Autodesk Inventor part; units mm, degrees
ref_plane "YZ Plane" through (0, 0, 0) normal (1, 0, 0) x (0, 1, 0)
ref_plane "XZ Plane" through (0, 0, 0) normal (0, 1, 0) x (-1, 0, 0)
ref_plane "XY Plane" through (0, 0, 0) normal (0, 0, 1) x (1, 0, 0)
sketch "Sketch1" plane through (0, 0, 0) normal (0, 0, 1) x (1, 0, 0)
  line L0 (-300, -400) -> (300, -400)
  line L1 (300, -400) -> (300, 400)
  line L2 (300, 400) -> (-300, 400)
  line L3 (-300, 400) -> (-300, -400)
  line L4 (-300, -400) -> (300, 400) construction
  line L5 (300, -400) -> (-300, 400) construction
  line L6 (-80, 360) -> (80, 360)
  line L7 (80, 360) -> (80, 400)
  line L8 (80, 400) -> (-80, 400)
  line L9 (-80, 400) -> (-80, 360)
  line L10 (-80, 360) -> (80, 400) construction
  line L11 (80, 360) -> (-80, 400) construction
  line L12 (-300, 280) -> (-260, 280)
  line L13 (-260, 280) -> (-180, 360)
  line L14 (-180, 360) -> (-180, 400)
  line L15 (180, 400) -> (180, 360)
  line L16 (180, 360) -> (260, 280)
  line L17 (260, 280) -> (300, 280)
  line L18 (-300, -275) -> (-260, -275)
  line L19 (-260, -275) -> (-260, -400)
  line L20 (300, -280) -> (260, -280)
  line L21 (260, -280) -> (260, -400)
  line L22 (0, 0) -> (0, 380) construction
  line L23 (-1, 360) -> (1, 360)
  line L24 (1, 360) -> (1, -400)
  line L25 (1, -400) -> (-1, -400)
  line L26 (-1, -400) -> (-1, 360)
  line L27 (-179, 400) -> (-179, 359.5858)
  line L28 (-179, 359.5858) -> (-259.5858, 279)
  line L29 (-259.5858, 279) -> (-300, 279)
  line L30 (-81, 359) -> (81, 359)
  line L31 (81, 359) -> (81, 401)
  line L32 (81, 401) -> (-81, 401)
  line L33 (-81, 401) -> (-81, 359)
  line L34 (-299, 399) -> (299, 399)
  line L35 (299, 399) -> (299, -399)
  line L36 (299, -399) -> (-299, -399)
  line L37 (-299, -399) -> (-299, 399)
  line L38 (-300, -274) -> (-259, -274)
  line L39 (-259, -274) -> (-259, -400)
  line L40 (259, -400) -> (259, -279)
  line L41 (259, -279) -> (300, -279)
  line L42 (300, 279) -> (259.5858, 279)
  line L43 (259.5858, 279) -> (179, 359.5858)
  line L44 (179, 359.5858) -> (179, 400)
  line L45 (-40, 360) -> (40, 360)
  line L46 (40, 360) -> (40, 280)
  line L47 (40, 280) -> (-40, 280)
  line L48 (-40, 280) -> (-40, 360)
  line L49 (-41, 361) -> (41, 361)
  line L50 (41, 361) -> (41, 279)
  line L51 (41, 279) -> (-41, 279)
  line L52 (-41, 279) -> (-41, 361)
  point P0 (-299, 279)
  point P1 (-299, -274)
  point P2 (-259, -399)
  point P3 (-1, -399)
  point P4 (-1, 359)
  point P5 (-81, 399)
  point P6 (-179, 399)
  point P7 (-1, 279)
  point P8 (-41, 359)
  dimension "d0" = 600
  dimension "d1" = 800
  dimension "d2" = 160
  dimension "d3" = 40
  dimension "d4" = 40
  dimension "d5" = 40
  dimension "d6" = 40
  dimension "d7" = 40
  dimension "d8" = 40
  dimension "d9" = 40
  dimension "d10" = 120
  dimension "d11" = 120
  dimension "d12" = 120
  dimension "d13" = 120
  dimension "d14" = 125
  dimension "d15" = 120
  dimension "d16" = 2
  dimension "d17" = 1
  dimension "d18" = 1
  dimension "d19" = 1
  dimension "d20" = 1
  dimension "d21" = 1
  dimension "d22" = 1
  dimension "d25" = 80
  dimension "d26" = 80
  dimension "d27" = 1
extrude "Extrusion1" add sketch "Sketch1" along normal blind 4 contours L39 L38 L37 L29 L28 L27 L34 L33 L30 L52 L51 L26 L36
fillet "Fillet1" radius 4 13 edges at (-179, 399, 2) (-179, 359.5858, 2) (-259.5858, 279, 2) (-299, 279, 2) (-81, 399, 2) (-81, 359, 2) (-41, 359, 2) (-41, 279, 2) (-1, 279, 2) (-1, -399, 2) (-259, -399, 2) (-259, -274, 2) (-299, -274, 2)
sketch "Sketch2" plane through (0, 0, 4) normal (0, 0, 1) x (1, 0, 0)
  arc A0 (-299, -270) -> (-295, -274) centre (-295, -270) ccw
  line L0 (-295, -274) -> (-263, -274)
  arc A1 (-259, -278) -> (-263, -274) centre (-263, -278) ccw
  line L1 (-259, -278) -> (-259, -395)
  arc A2 (-259, -395) -> (-255, -399) centre (-255, -395) ccw
  line L2 (-255, -399) -> (-5, -399)
  arc A3 (-5, -399) -> (-1, -395) centre (-5, -395) ccw
  line L3 (-1, -395) -> (-1, 275)
  arc A4 (-1, 275) -> (-5, 279) centre (-5, 275) ccw
  line L4 (-5, 279) -> (-37, 279)
  arc A5 (-41, 283) -> (-37, 279) centre (-37, 283) ccw
  line L5 (-41, 283) -> (-41, 355)
  arc A6 (-41, 355) -> (-45, 359) centre (-45, 355) ccw
  line L6 (-45, 359) -> (-77, 359)
  arc A7 (-81, 363) -> (-77, 359) centre (-77, 363) ccw
  line L7 (-81, 363) -> (-81, 395)
  arc A8 (-81, 395) -> (-85, 399) centre (-85, 395) ccw
  line L8 (-85, 399) -> (-175, 399)
  arc A9 (-175, 399) -> (-179, 395) centre (-175, 395) ccw
  line L9 (-179, 395) -> (-179, 361.2426)
  arc A10 (-180.1716, 358.4142) -> (-179, 361.2426) centre (-183, 361.2426) ccw
  line L10 (-180.1716, 358.4142) -> (-258.4142, 280.1716)
  arc A11 (-261.2426, 279) -> (-258.4142, 280.1716) centre (-261.2426, 283) ccw
  line L11 (-261.2426, 279) -> (-295, 279)
  arc A12 (-295, 279) -> (-299, 275) centre (-295, 275) ccw
  line L12 (-299, 275) -> (-299, -270)
  line L13 (-170, 358) -> (-90, 358)
  line L14 (-90, 358) -> (-90, 278)
  line L15 (-90, 278) -> (-170, 278)
  line L16 (-170, 278) -> (-170, 358)
  line L17 (-170, 358) -> (-90, 278) construction
  line L18 (-90, 358) -> (-170, 278) construction
  line L19 (-130, 318) -> (-130, 358) construction
  line L20 (-170, 358) -> (-175, 395) construction
  line L21 (-90, 358) -> (-85, 395) construction
  line L22 (-165.75, 282.25) -> (-94.25, 282.25) construction
  line L23 (-94.25, 282.25) -> (-94.25, 353.75) construction
  line L24 (-94.25, 353.75) -> (-165.75, 353.75) construction
  line L25 (-165.75, 353.75) -> (-165.75, 282.25) construction
  line L26 (-165.75, 282.25) -> (-94.25, 353.75) construction
  line L27 (-94.25, 282.25) -> (-165.75, 353.75) construction
  circle A13 centre (-165.75, 353.75) radius 2.5
  circle A14 centre (-94.25, 353.75) radius 2.5
  circle A15 centre (-94.25, 282.25) radius 2.5
  circle A16 centre (-165.75, 282.25) radius 2.5
  circle A17 centre (-165.75, 353.75) radius 6.5
  line L28 (-165.75, 347.25) -> (-170, 347.25)
  line L29 (-159.25, 353.75) -> (-159.25, 358)
  circle A18 centre (-165.75, 282.25) radius 6.5
  line L30 (-165.75, 288.75) -> (-170, 288.75)
  line L31 (-159.25, 282.25) -> (-159.25, 278)
  circle A19 centre (-94.25, 282.25) radius 6.5
  line L32 (-100.75, 282.25) -> (-100.75, 278)
  line L33 (-94.25, 288.75) -> (-90, 288.75)
  circle A20 centre (-94.25, 353.75) radius 6.5
  line L34 (-94.25, 347.25) -> (-90, 347.25)
  line L35 (-100.75, 353.75) -> (-100.75, 358)
  point P0 (0, 0)
  point P1 (-100.75, 358)
  point P2 (-170, 288.75)
  point P3 (-100.75, 278)
  point P4 (-90, 288.75)
  point P5 (-90, 347.25)
  dimension "d29" = 80
  dimension "d30" = 80
  dimension "d31" = 41
  dimension "d32" = 71.5
  dimension "d33" = 71.5
  dimension "d34" = 5
  dimension "d35" = 5
  dimension "d36" = 5
  dimension "d37" = 5
  dimension "d38" = 4
  dimension "d41" = 360
extrude "Extrusion2" cut sketch "Sketch2" against normal blind 4 contours L13 L35 A20 L34 L14 L33 A19 L32 L15 L31 A18 L30 L16 L28 A17 L29 | A13 | A14 | A15 | A16
fillet "Fillet2" radius 4 8 edges at (-100.75, 358, 2) (-90, 347.25, 2) (-90, 288.75, 2) (-100.75, 278, 2) (-159.25, 358, 2) (-170, 347.25, 2) (-170, 288.75, 2) (-159.25, 278, 2)
properties part number "RT_FRM_MC_014_FrontCover_L" material "Polycarbonate, Smoke"
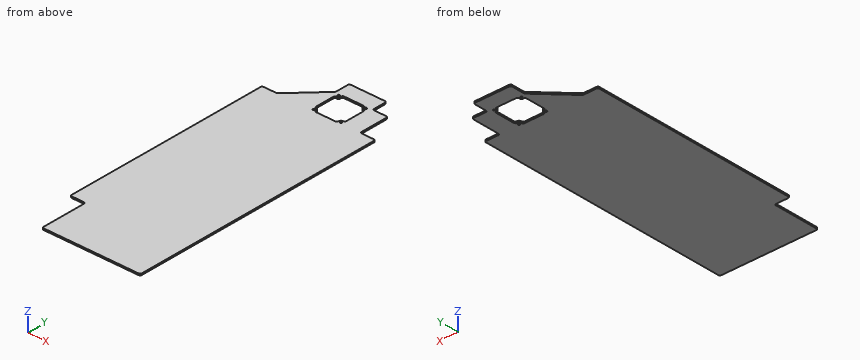
Input: part model. Units: mm. Frame: model coordinates. Give positions to 0.01 mm unless a question says otherwise; leave off trailing zeros. Loops run counter-clockwise (first coordinate to the right, second up) from the corner with the lowest first, then second, coordinate; pieces in that order, holes last. Notation, with made-up numbers: M 16,-40 L 28,-40 A12 ccw 28,-27 Z; hole C -24,33 d6. An arc over 180 degrees is marked long. Use CSV: the item, a comma, the result in double quotes.
(1) Section B-B, the plane x = -69. Return loops of the section in (y, z).
Outcome:
outline,"M -399,0 L 359,0 L 359,4 L -399,4 Z"
(2) Section A-A, the plane z = 2.9. Count the separate pieces of the cut face and the enclosed holes in it, plus the area to 3 significant figures.
Outcome:
separate pieces,"1"
enclosed holes,"5"
area,"209,000 mm²"
(3) Material intervals for L1, parallel to Y at x = -165.75, z = 2.4; L2, parallel to Y at x = -108, z = 3.5, sorted ascending. Write a range as [from, to].
Outcome:
L1,"y = [-399, 279.75], [284.75, 288.75], [347.25, 351.25], [356.25, 399]"
L2,"y = [-399, 278], [358, 399]"
(4) Pin query (flat end, axial travel): P1, Ø1.2, axis at y = -361, z = 1, coming from the -X side; P2, Ø1.2, axis at x = -13.5, z = 1, coming from the +Y side; P3, Ø1.2, axis at x = -284.5, z = 2.5, coming from the -Y side. Return the tip coordinate at first contact, or that it passes through.
Outcome:
P1,"stops at x = -259"
P2,"stops at y = 279"
P3,"stops at y = -274"
(5) Section C-C, the plane x = -194. Return loops of the section in (y, z).
Outcome:
outline,"M -399,0 L 344.59,0 L 344.59,4 L -399,4 Z"
